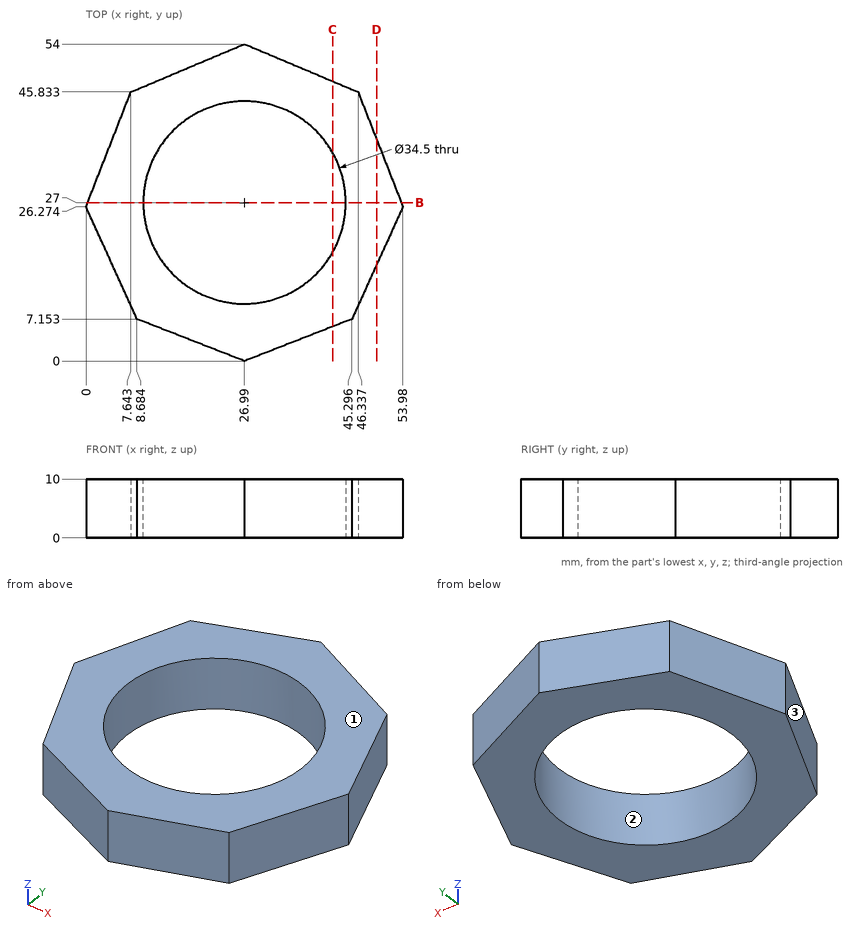
Study the drawing (mm; zero at the part's minimum x, y, z) and answer. Coordinates: 2 decimals unless noted, no trailing zeros. Order: outer loops, then holes, each group sorted by start corner. A loop starts at its lowest first (then second) coordinate and runs counter-clockwise, first axis right, second up. Notation, with made-up numbers: M 48.5,-28.5 L 95.5,-28.5 A21 ccw 95.5,-24.5 Z; hole C 62,62.25 d11. An arc over 180 degrees is marked long. Answer as a JSON object with one key per item and string values. Group by question number.
1. Determine the mould class of the marked faces 1, 2 and 3 for opening direction Y: released by +Y, released by -Y, zero draft, split by the parting line, or undercut.
2. Flat-ended cylindrical pins translate along their axes: P1, Ø6, axis at y = 33.5, z = 4, coming from the -X side; P2, Ø6, axis at x = 18, z = 7, coming from the -Y side; P3, Ø2, axis at y = 41.5, z = 9, coming from the -X side. Find the tip coordinate at first contact, or state that the pin passes through.
3. Straight lines are drawn through the part: line 1 (Y direction, x = 40.5, z = 4.5) (1 decimal); line 2 (X direction, y = 30, z = 4) (1 decimal); line 3 (X direction, y = 37.5, z = 5.5) (1 decimal). For each, find the intervals that lie inside material, in ascending order.
4. Section B-B on y = 27 is taken. Write down the section's boundary in (x, z).
5. Section D-D on x = 49.5 is taken. Write down the section's boundary in (y, z).
6. Section C-C on x = 42 is taken. Write down the section's boundary in (y, z) (1 decimal).
Values follow:
{
 "1": {"face 1": "zero draft", "face 2": "undercut", "face 3": "released by -Y"},
 "2": {"P1": "x = 1.65", "P2": "y = 2.34", "P3": "x = 5.56"},
 "3": {"line 1": "5.3 to 16.3, 37.7 to 48.3", "line 2": "1.5 to 10, 44 to 52.5", "line 3": "4.4 to 13.3, 40.7 to 49.6"},
 "4": {"outline": "M 0.28,0 L 9.74,0 L 9.74,10 L 0.28,10 Z; M 44.24,0 L 53.7,0 L 53.7,10 L 44.24,10 Z"},
 "5": {"outline": "M 16.41,0 L 37.74,0 L 37.74,10 L 16.41,10 Z"},
 "6": {"outline": "M 5.9,0 L 18.5,0 L 18.5,10 L 5.9,10 Z; M 35.5,0 L 47.7,0 L 47.7,10 L 35.5,10 Z"}
}
